from build123d import *


with BuildPart() as part:
    # Sketch1 → Revolve1 (revolve)
    with BuildSketch(Plane.XY):
        Polygon((-9, 7.35), (-13, 7.35), (-13, -0.95), (-14.8, -0.95), (-15, -1.15), (-15, -7.75), (-11, -7.75), (-11, -6.25), (-11.75, -6.25), (-11.75, -5.25), (-11, -5.25), (-11, 5.25), (-9, 5.25), align=None)
    revolve(axis=Axis((0, 0, 0), (0, -1, 0)))


solid = part.part
Here's how the part is built. I have some questions about the finished solid (model axes, mm). A direction names the side the tool comes from. Give positions to 0.01 mm unless a question says otherwise; leave off trailing zeros. Order: outer loops, then holes, each group sorted by start corner. A loop starts at its lowest first (then second) coordinate and runs counter-clockwise, first axis right, second up. Notation, with made-up numbers: (31.25, 82) -> (84.25, 82) arc R17 ccw to (84.25, 105) -> close; hole circle Ø9 at (58.5, 78). An arc over 180 degrees is marked (long way). One line per item, written item: value. Start each with the question number.
1. For faces 1 (the face through (2.38, 0.07, 10.74)), 2 (the face through (-8, -5.25, 8)), 3 (the face through (1.172, 6.315, -8.923)), which set-ups out of +Z, -Z, +X, -X, +Y, -Y let a thin tool reach every point of the face, with its end or its side?
2. I need wall thicknesses on probe 1 along X at (y, z) = (-5.8, 0); probe 2 along Z at (x, y) = (0, 5.95). Which ranges of each line are inside material? Lowest first, please. Write a range as from..to.
3. Imagine slicing it at D-D, the plane y = 0.25. List the corners of the cut face in (x, z) for me.
4. Imagine slicing it at C-C, the plane y = 6.25. List the corners of the cut face in (x, z) for me.
5. Imagine slicing it at A-A, the plane x = 0. List the corners of the cut face in (y, z) for me, plus the area to 3 significant figures.
6. Imagine slicing it at B-B, the plane z = 0. List the corners of the cut face in (x, y) for me, plus the area to 3 significant figures.
7. Will these pins go through, and if not, where does the flat tip stop? pin 1 Ø4 at (x, y) = (-4, -1.5) entering from +Z; pin 2 Ø2 at (x, z) = (0, 7.5) entering from +Y; pin 3 Ø1.5 at (x, y) = (5.5, 0) entering from +Z; pin 4 Ø8 at (x, y) = (1, 3) entering from -Z.
8. We'd pull the mould along Z, two halves only. Please class faces 4 (the face through (8, -6.25, 8)), 5 (the face through (9, -0.95, 10)), 6 (the face through (10.316, 3.142, 7.91)), 7 (the face through (2.38, -6.99, 10.74)): released by +Z, released by -Z, zero draft, split by the parting line, or undercut.
Values follow:
1. face 1: -Y
1. face 2: none
1. face 3: +Y, -Y
2. probe 1: x = -15..-11.75, 11.75..15
2. probe 2: z = -13..-9, 9..13
3. outline: circle Ø26 at (0, 0); hole circle Ø22 at (0, 0)
4. outline: circle Ø26 at (0, 0); hole circle Ø18 at (0, 0)
5. outline: (-7.75, -15) -> (-1.15, -15) -> (-0.95, -14.8) -> (-0.95, -13) -> (7.35, -13) -> (7.35, -9) -> (5.25, -9) -> (5.25, -11) -> (-5.25, -11) -> (-5.25, -11.75) -> (-6.25, -11.75) -> (-6.25, -11) -> (-7.75, -11) -> close; (-7.75, 11) -> (-6.25, 11) -> (-6.25, 11.75) -> (-5.25, 11.75) -> (-5.25, 11) -> (5.25, 11) -> (5.25, 9) -> (7.35, 9) -> (7.35, 13) -> (-0.95, 13) -> (-0.95, 14.8) -> (-1.15, 15) -> (-7.75, 15) -> close
5. area: 94.5 mm2
6. outline: (-15, -7.75) -> (-11, -7.75) -> (-11, -6.25) -> (-11.75, -6.25) -> (-11.75, -5.25) -> (-11, -5.25) -> (-11, 5.25) -> (-9, 5.25) -> (-9, 7.35) -> (-13, 7.35) -> (-13, -0.95) -> (-14.8, -0.95) -> (-15, -1.15) -> close; (9, 5.25) -> (11, 5.25) -> (11, -5.25) -> (11.75, -5.25) -> (11.75, -6.25) -> (11, -6.25) -> (11, -7.75) -> (15, -7.75) -> (15, -1.15) -> (14.8, -0.95) -> (13, -0.95) -> (13, 7.35) -> (9, 7.35) -> close
6. area: 94.5 mm2
7. pin 1: stops at z = 14.87
7. pin 2: passes through
7. pin 3: stops at z = 12.1
7. pin 4: stops at z = -14.82
8. face 4: undercut
8. face 5: zero draft
8. face 6: split by the parting line
8. face 7: undercut
